Design review of the part built by this model. Coordinates are the model's own, in mm. Face numbers are marked on the shaded views. A direction names the side the tool comes from. Give positions to 0.01 mm unless a question says otherwise; leave off trailing zeros. Write each loop counter-clockwise with the first axis right and the second up, starting at its lowest first coordinate (ties: lowest second). Pieces come first, ordered by that corner, then holes. Notation, with made-up numbers: (5, 17.5) - (29, 17.5) arc R20 ccw to (29, 21.5) - close; hole circle Ø2 at (56.5, 16.25). An arc over 180 degrees is marked (long way). Use a Markdown table: item, result. Add a question column.
```python
from build123d import *

# Parameters (mm, degrees)
RESSALTO_EXTRUS_O1_DEPTH      = 15
RESSALTO_EXTRUS_O1_DEPTH_BACK = 15
ESBO_O2_W                     = 20
ESBO_O2_H                     = 6.210978077
RESSALTO_EXTRUS_O2_DEPTH      = 12
RESSALTO_EXTRUS_O3_START      = -20
RESSALTO_EXTRUS_O3_DEPTH      = 20
CORTE_EXTRUS_O1_START         = -3.8
ESBO_O6_W                     = 3
ESBO_O6_H                     = 6
CORTE_EXTRUS_O1_DEPTH         = 3.8
ESBO_O7_W                     = 14.512469108
ESBO_O7_H                     = 20
RESSALTO_EXTRUS_O4_DEPTH      = 3


with BuildPart() as part:
    # Esboço1 → Ressalto-extrusão1 (new, two sides: drawn at the far end of the back side and taken through both)
    with BuildSketch(Plane.XY.offset(-RESSALTO_EXTRUS_O1_DEPTH_BACK)):
        with BuildLine():
            Line((0, 16.196411572), (0, 11.255433495))
            Line((0, 11.255433495), (20.3764132, 1.849909993))
            Line((20.3764132, 1.849909993), (39.444832225, -16.570361831))
            Line((39.444832225, -16.570361831), (49.347871005, -19.041211572))
            Line((49.347871005, -19.041211572), (52.316343324, -17.041005068))
            ThreePointArc((52.316343324, -17.041005068), (52.649617834, -16.475732), (52.419959407, -15.861026747))
            Line((52.419959407, -15.861026747), (29.43843308, 6.339343474))
            Line((29.43843308, 6.339343474), (2.234792117, 18.89623864))
            ThreePointArc((2.234792117, 18.89623864), (0.726083483, 18.792939111), (0, 17.466411572))
            Line((0, 17.466411572), (0, 16.196411572))
        make_face()
    extrude(amount=RESSALTO_EXTRUS_O1_DEPTH + RESSALTO_EXTRUS_O1_DEPTH_BACK)

    # Esboço2 → Ressalto-extrusão2 (add)
    with BuildSketch(Plane.ZY):
        with Locations((0, 14.360922534)):
            Rectangle(ESBO_O2_W, ESBO_O2_H)
    extrude(amount=RESSALTO_EXTRUS_O2_DEPTH)

    # Esboço4 → Ressalto-extrusão3 (add)
    with BuildSketch(Plane.XY.offset(10).offset(RESSALTO_EXTRUS_O3_START)):
        Polygon((-4.5, 11.255433495), (-1.5, 11.255433495), (-1.5, 6.255433495), (-0.7, 6.255433495), (-0.7, 6.015731828), (-1.5, 5.255433495), (-4.5, 5.255433495), align=None)
    extrude(amount=RESSALTO_EXTRUS_O3_DEPTH)

    # Esboço6 → Corte-extrusão1 (cut)
    with BuildSketch(Plane.ZY.offset(4.5).offset(CORTE_EXTRUS_O1_START)):
        with Locations((-8.5, 8.255433495)):
            Rectangle(ESBO_O6_W, ESBO_O6_H)
        with Locations((8.5, 8.255433495)):
            Rectangle(ESBO_O6_W, ESBO_O6_H)
    extrude(amount=CORTE_EXTRUS_O1_DEPTH, mode=Mode.SUBTRACT)

    # Esboço7 → Ressalto-extrusão4 (add)
    with BuildSketch(Plane(origin=(10.760423423, 11.139046409, 0), x_dir=(0.7192245636353503, -0.6947776817540559, 0), z_dir=(-0.6947776817540559, -0.7192245636353503, 0))):
        with Locations((26.62617527, 0)):
            Rectangle(ESBO_O7_W, ESBO_O7_H)
    extrude(amount=RESSALTO_EXTRUS_O4_DEPTH)


solid = part.part
```
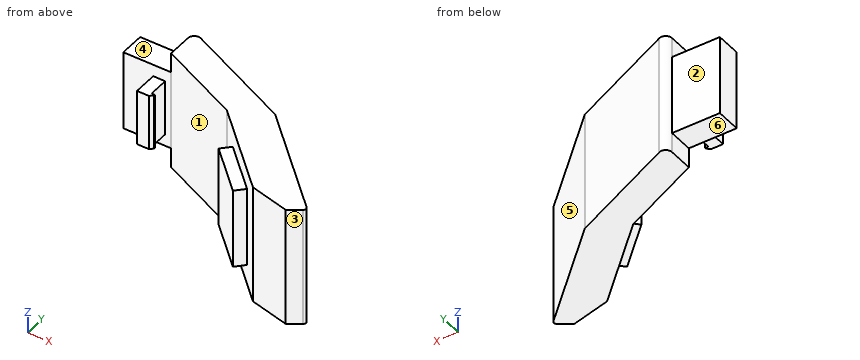
(1) Insertion check: pin 1 (1.1 mm diameter, centred on x = -3.5, y = 8, fed in from -Z); pin 2 (1.8 mm diameter, centred on y = 7, z = -3, fed in from -X); pin 3 (1 mm diameter, centred on x = 39.5, z = 9, fed in from +Y); pin 4 (10 mm diameter, centred on y = -12.5, z = -3.5, fed in from +X). Each pin has a flat end and moves straight along its axis. Give the tip position at first contact, or say it passes through.
(2) For line 1 along Z through (x, y) = (-2.5, 11); line 2 along X through (y, z) = (17, 6.75); line 3 along X through (y, z) = (-13, 1.25), list the stretches that pass through material, from the lowest coordinate up.
(3) Add section D-D (z = -1.75). State the section outline as (x, y) points, and give its area (3 significant figures).
(4) Mouldability with a two-part tool opening along X and no side actions: class the marked faces 1, 2 and 3 as +X half, -X half, draft (parallel to the pull), parting line (faces both ways), or undercut.
(5) Add section B-B (y = -6.5). State the section outline as (x, z) points.
(6) Add section C-C (x = 41). State the section outline as (y, z) points.
(7) Tool access review of the marked faces 4, 5 and 6: name each direction out of +Z, -Z, +X, -X, +Y, -Y from which nothing blocks a thin tool from reaching the whole face with its end or side.
(8) Add section A-A (z = 13.25). State the section outline as (x, y) points.
Answers follow:
| question | item | result |
|---|---|---|
| 1 | pin 1 | z = -7 |
| 1 | pin 2 | x = -4.5 |
| 1 | pin 3 | y = -2.9 |
| 1 | pin 4 | x = 52.65 |
| 2 | line 1 | -7 to 7 |
| 2 | line 2 | -12 to 6.34 |
| 2 | line 3 | 31.43 to 34.55, 35.75 to 49.46 |
| 3 | outline | (-12, 11.26) - (-4.5, 11.26) - (-4.5, 5.26) - (-1.5, 5.26) - (-0.7, 6.02) - (-0.7, 6.26) - (-1.5, 6.26) - (-1.5, 11.26) - (0, 11.26) - (20.38, 1.85) - (24.69, -2.32) - (22.61, -4.48) - (33.05, -14.56) - (35.13, -12.4) - (39.44, -16.57) - (49.35, -19.04) - (52.32, -17.04) arc R0.76 ccw to (52.42, -15.86) - (29.44, 6.34) - (2.23, 18.9) arc R1.57 ccw to (0, 17.47) - (-12, 17.47) - close |
| 3 | area | 651 mm^2 |
| 4 | face 1 | undercut |
| 4 | face 2 | draft |
| 4 | face 3 | +X half |
| 5 | outline | (24.7, -10) - (29.02, -10) - (29.02, -15) - (42.73, -15) - (42.73, 15) - (29.02, 15) - (29.02, 10) - (24.7, 10) - close |
| 6 | outline | (-16.96, -15) - (-4.83, -15) - (-4.83, 15) - (-16.96, 15) - close |
| 7 | face 4 | +Z, -X, +Y, -Y |
| 7 | face 5 | +Z, -Z, +X, +Y |
| 7 | face 6 | -Z, -X, +Y, -Y |
| 8 | outline | (0, 11.26) - (20.38, 1.85) - (39.44, -16.57) - (49.35, -19.04) - (52.32, -17.04) arc R0.76 ccw to (52.42, -15.86) - (29.44, 6.34) - (2.23, 18.9) arc R1.57 ccw to (0, 17.47) - close |
